```python
from build123d import *

# Parameters (mm, degrees)
SKETCH1_W           = 55
SKETCH1_H           = 55
BOSS_EXTRUDE1_DEPTH = 3
SKETCH2_W           = 10
SKETCH2_H           = 3
SKETCH2_W_2         = 15
CUT_EXTRUDE1_DEPTH  = 3
SKETCH3_W           = 55
SKETCH3_H           = 30
BOSS_EXTRUDE2_DEPTH = 3
SKETCH4_W           = 144
SKETCH4_H           = 52
BOSS_EXTRUDE3_DEPTH = 3
SKETCH5_W           = 199
SKETCH5_H           = 13
BOSS_EXTRUDE4_DEPTH = 3
SKETCH6_W           = 199
SKETCH6_H           = 20
BOSS_EXTRUDE5_DEPTH = 3
SKETCH7_R           = 2
SKETCH7_W           = 40
SKETCH7_H           = 20
CUT_EXTRUDE22_DEPTH = 33
SKETCH8_W           = 40
SKETCH8_H           = 9
CUT_EXTRUDE23_DEPTH = 33
SKETCH9_W           = 63.816090929
SKETCH9_H           = 30.906314682
BOSS_EXTRUDE6_DEPTH = 3


with BuildPart() as part:
    # Sketch1 → Boss-Extrude1 (new body)
    with BuildSketch(Plane.XY):
        Rectangle(SKETCH1_W, SKETCH1_H)
    extrude(amount=BOSS_EXTRUDE1_DEPTH)

    # Sketch2 → Cut-Extrude1 (cut)
    with BuildSketch(Plane.XY.offset(3)):
        with Locations((22.5, -26)):
            Rectangle(SKETCH2_W, SKETCH2_H)
        with Locations((2.5, -26)):
            Rectangle(SKETCH2_W, SKETCH2_H)
        with Locations((-20, -26)):
            Rectangle(SKETCH2_W_2, SKETCH2_H)
    extrude(amount=-CUT_EXTRUDE1_DEPTH, mode=Mode.SUBTRACT)

    # Sketch3 → Boss-Extrude2 (add)
    with BuildSketch(Plane(origin=(0, 0, 0), x_dir=(-1, 0, 0), z_dir=(0, 0, -1))):
        with Locations((0, -42.5)):
            Rectangle(SKETCH3_W, SKETCH3_H)
    extrude(amount=-BOSS_EXTRUDE2_DEPTH)

    # Sketch4 → Boss-Extrude3 (add)
    with BuildSketch(Plane(origin=(0, 0, 0), x_dir=(-1, 0, 0), z_dir=(0, 0, -1))):
        with Locations((99.5, 1.5)):
            Rectangle(SKETCH4_W, SKETCH4_H)
    extrude(amount=-BOSS_EXTRUDE3_DEPTH)

    # Sketch5 → Boss-Extrude4 (add)
    with BuildSketch(Plane(origin=(0, 0, 0), x_dir=(-1, 0, 0), z_dir=(0, 0, -1))):
        with Locations((72, 34)):
            Rectangle(SKETCH5_W, SKETCH5_H)
    extrude(amount=-BOSS_EXTRUDE4_DEPTH)

    # Sketch6 → Boss-Extrude5 (add)
    with BuildSketch(Plane(origin=(0, 0, 0), x_dir=(-1, 0, 0), z_dir=(0, 0, -1))):
        with Locations((72, 50.5)):
            Rectangle(SKETCH6_W, SKETCH6_H)
    extrude(amount=-BOSS_EXTRUDE5_DEPTH)

    # Sketch7 → Cut-Extrude22 (cut)
    with BuildSketch(Plane(origin=(0, 0, 0), x_dir=(-1, 0, 0), z_dir=(0, 0, -1))):
        with Locations((168.5, 46.5)):
            Circle(SKETCH7_R)
        with Locations((168.5, 36.5)):
            Circle(SKETCH7_R)
        with Locations((118.5, 36.5)):
            Circle(SKETCH7_R)
        with Locations((118.5, 46.5)):
            Circle(SKETCH7_R)
        with Locations((143.5, 41.5)):
            Rectangle(SKETCH7_W, SKETCH7_H)
    extrude(amount=-CUT_EXTRUDE22_DEPTH, mode=Mode.SUBTRACT)

    # Sketch8 → Cut-Extrude23 (cut)
    with BuildSketch(Plane(origin=(0, 0, 0), x_dir=(-1, 0, 0), z_dir=(0, 0, -1))):
        with Locations((143.5, 56)):
            Rectangle(SKETCH8_W, SKETCH8_H)
    extrude(amount=-CUT_EXTRUDE23_DEPTH, mode=Mode.SUBTRACT)

    # Sketch9 → Boss-Extrude6 (add)
    with BuildSketch(Plane(origin=(0, 0, 0), x_dir=(-1, 0, 0), z_dir=(0, 0, -1))):
        with Locations((139.591954536, 45.046842659)):
            Rectangle(SKETCH9_W, SKETCH9_H)
    extrude(amount=-BOSS_EXTRUDE6_DEPTH)


solid = part.part
```
Source: CAD feature listing. Evaluate the final solid. Frame: model axes, mm. Coordinates: 2 decimals unless noted, no trailing zeros. Loops run counter-clockwise (first coordinate to the right, second up) from the corner with the lowest first, then second, coordinate; pieces in that order, holes last. Notation, with made-up numbers: M 55,77 L 90,77 A12 ccw 90,100 Z; hole C 66,52.25 d4. An arc over 180 degrees is marked long. Put each result on its own line as item: value. Start each with the question number.
1) Cut plane B-B on z = 1.3. Return the cut outline in (x, y).
2) Cut plane A-A on x = -19. Return the cut outline in (y, z), then the cut area to 3 significant figures.
3) Cut plane C-C on y = -46.5. Return the cut outline in (x, z).
4) Contact query for flat-ended pins moving along their axis: pin 1 Ø0.9 at (x, z) = (-126.5, 1) entering from -Y; pin 2 Ø0.9 at (y, z) = (-26, 2) entering from +X; pin 3 Ø1.5 at (y, z) = (-26.5, 2) entering from -X; pin 4 Ø10 at (x, y) = (-15, 24.5) entering from -Z. Output: stop coordinate, or through.
5) Ray query, L1, parallel to Y at x = -92.5, z = 0.3; L2, parallel to X at y = -33, z = 1.4. Return the intervals inside material, ascending. Write a range as from..to.
6) Cut plane D-D on x = -74.5. Return the cut outline in (y, z).
The answers:
1. outline: M -171.5,-24.5 L -12.5,-24.5 L -12.5,-27.5 L -27.5,-27.5 L -27.5,-57.5 L 27.5,-57.5 L 27.5,-27.5 L 17.5,-27.5 L 17.5,-24.5 L 27.5,-24.5 L 27.5,60.5 L -171.5,60.5 Z; hole M -2.5,-27.5 L 7.5,-27.5 L 7.5,-24.5 L -2.5,-24.5 Z
2. outline: M -57.5,0 L -27.5,0 L -27.5,3 L -57.5,3 Z; M -24.5,0 L 60.5,0 L 60.5,3 L -24.5,3 Z
2. area: 345 mm²
3. outline: M -27.5,0 L 27.5,0 L 27.5,3 L -27.5,3 Z
4. pin 1: stops at y = -24.5
4. pin 2: stops at x = 17.5
4. pin 3: stops at x = -12.5
4. pin 4: stops at z = 0
5. L1: y = -24.5..60.5
5. L2: x = -27.5..27.5
6. outline: M -24.5,0 L 60.5,0 L 60.5,3 L -24.5,3 Z
